Source: CAD feature listing. Evaluate the final solid. Frame: model axes, mm. A direction names the side the tool comes from. Coordinates: 2 decimals unless noted, no trailing zeros. Loops run counter-clockwise (first coordinate to the right, second up) from the corner with the lowest first, then second, coordinate; pieces in that order, holes last. Notation, with made-up numbers: (34.5, 3) -> (75.5, 3) arc R25 cw to (75.5, 19) -> close; hole circle Ø7 at (13, 19.25). An arc over 180 degrees is marked (long way). Answer as CSV lines item,"result".
from build123d import *

# Parameters (mm, degrees)
SKETCH1_W           = 260
SKETCH1_H           = 255
SKETCH1_R           = 60
BOSS_EXTRUDE1_DEPTH = 8
SKETCH2_W           = 315
SKETCH2_H           = 70
SKETCH2_W_2         = 80
SKETCH2_H_2         = 30
SKETCH2_W_3         = 70
BOSS_EXTRUDE2_DEPTH = 60
BOSS_EXTRUDE3_DEPTH = 60
CUT_EXTRUDE1_REACH  = 282.827
CUT_EXTRUDE2_REACH  = 282.827


with BuildPart() as part:
    # Sketch1 → Boss-Extrude1 (new body)
    with BuildSketch(Plane.XY):
        with Locations((130, 127.5)):
            Rectangle(SKETCH1_W, SKETCH1_H)
        with Locations((130, 145)):
            Circle(SKETCH1_R, mode=Mode.SUBTRACT)
    extrude(amount=BOSS_EXTRUDE1_DEPTH)

    # Sketch2 → Boss-Extrude2 (add)
    with BuildSketch(Plane.XY.offset(8)):
        with Locations((130, -35)):
            Rectangle(SKETCH2_W, SKETCH2_H)
        with Locations((40, -35)):
            Rectangle(SKETCH2_W_2, SKETCH2_H_2, mode=Mode.SUBTRACT)
        with Locations((220, -35)):
            Rectangle(SKETCH2_W_2, SKETCH2_H_2, mode=Mode.SUBTRACT)
        with Locations((130, -35)):
            Rectangle(SKETCH2_W_3, SKETCH2_H_2, mode=Mode.SUBTRACT)
    extrude(amount=-BOSS_EXTRUDE2_DEPTH)

    # Sketch3 → Boss-Extrude3 (add)
    with BuildSketch(Plane(origin=(0, 0, 0), x_dir=(1, 0, 0), z_dir=(0, 1, 0))):
        Polygon((260, -8), (287.5, 42), (284.121880998, 43.857965451), (260, 0), align=None)
        Polygon((0, -8), (-27.5, 42), (-24.121880998, 43.857965451), (0, 0), align=None)
    extrude(amount=BOSS_EXTRUDE3_DEPTH)

    # Sketch4 → Cut-Extrude1 (cut, up to next)
    with BuildSketch(Plane(origin=(202.994241843, 0, 111.646833013), x_dir=(0.48191875, 0, -0.876215909), z_dir=(0.876215909, 0, 0.48191875)), mode=Mode.PRIVATE) as cut_extrude1_sk1:
        Polygon((175.352708724, 0), (125.298874941, 60), (175.352708724, 60), align=None)
    cut_extrude1_tool1 = extrude(cut_extrude1_sk1.sketch, amount=-CUT_EXTRUDE1_REACH, mode=Mode.PRIVATE) & part.part
    add(cut_extrude1_tool1.solids().sort_by_distance((279.459373, 40, -27.380678))[0], mode=Mode.SUBTRACT)

    # Sketch5 → Cut-Extrude2 (cut, up to next)
    with BuildSketch(Plane(origin=(-3.378119002, 0, 1.857965451), x_dir=(0.48191875, 0, 0.876215909), z_dir=(-0.876215909, 0, 0.48191875)), mode=Mode.PRIVATE) as cut_extrude2_sk1:
        Polygon((-50.053833783, 0), (0, 60), (-50.053833783, 60), align=None)
    cut_extrude2_tool1 = extrude(cut_extrude2_sk1.sketch, amount=-CUT_EXTRUDE2_REACH, mode=Mode.PRIVATE) & part.part
    add(cut_extrude2_tool1.solids().sort_by_distance((-19.459373, 40, -27.380678))[0], mode=Mode.SUBTRACT)


solid = part.part
(1) Cut plane A-A (y = 145). Return the cut outline in (x, z), then the cut area to 3 significant figures.
Computed values:
outline,"(0, 0) -> (70, 0) -> (70, 8) -> (0, 8) -> close; (190, 0) -> (260, 0) -> (260, 8) -> (190, 8) -> close"
area,"1,120 mm^2"
(2) Material intervals for L1, parallel to Y at x = 130, z = 4; L2, parallel to Y at x = 75, z = -24; L3, parallel to Y at x = 232.5, z = 1, sorted ascending. Write a range as [from, to].
Computed values:
L1,"[-70, -50], [-20, 85], [205, 255]"
L2,"[-70, -50], [-20, 0]"
L3,"[-70, -50], [-20, 255]"
(3) Cut plane D-D (z = -27). Return the cut outline in (x, y).
Computed values:
outline,"(-27.5, -70) -> (287.5, -70) -> (287.5, 0) -> (279.25, 0) -> (279.25, 20.52) -> (274.85, 23.06) -> (274.85, 0) -> (-14.85, 0) -> (-14.85, 23.06) -> (-19.25, 20.52) -> (-19.25, 0) -> (-27.5, 0) -> close; hole (0, -50) -> (80, -50) -> (80, -20) -> (0, -20) -> close; hole (95, -50) -> (165, -50) -> (165, -20) -> (95, -20) -> close; hole (180, -50) -> (260, -50) -> (260, -20) -> (180, -20) -> close"
(4) Pin query (flat end, axial travel): pin 1 Ø6.5 at (y, z) = (204.5, 5.5) entering from +X; pin 2 Ø6 at (x, z) = (27, -29.5) entering from +Y; pin 3 Ø14 at (x, z) = (268, -25) entering from +Y. Return the tip coordinate at first contact, or that it passes through.
Computed values:
pin 1,"x = 260"
pin 2,"y = 0"
pin 3,"y = 34.95"
(5) Cut plane C-C (x = 205). Return the cut outline in (y, z), then the cut area to 3 significant figures.
Computed values:
outline,"(-70, -52) -> (-50, -52) -> (-50, 8) -> (-70, 8) -> close; (-20, -52) -> (0, -52) -> (0, 0) -> (255, 0) -> (255, 8) -> (-20, 8) -> close"
area,"4,440 mm^2"
(6) Cut plane B-B (x = 130). Return the cut outline in (y, z).
Computed values:
outline,"(-70, -52) -> (-50, -52) -> (-50, 8) -> (-70, 8) -> close; (-20, -52) -> (0, -52) -> (0, 0) -> (85, 0) -> (85, 8) -> (-20, 8) -> close; (205, 0) -> (255, 0) -> (255, 8) -> (205, 8) -> close"
(7) Draft query along Y for faces 4 (the flat face through (-10.5, 22.91, -11.09)), 5 (the flat face through (-13.9, 29.6, -21.3)), 6 (the flat face through (180, -35, -22)). Return one class per face: released by +Y, released by -Y, zero draft, split by the parting line, or undercut.
Computed values:
face 4,"zero draft"
face 5,"released by +Y"
face 6,"undercut"
(8) Access query for faces 1 (the flat face through (219, -20, -22)), 2 (the flat face through (280, 0, -6)), 3 (the flat face through (-6.87, 16.25, -12.49)). Directions: +Z, -Z, +X, -X, +Y, -Y. A direction counts if a zero-diameter tool reaches every point of the face in a straight line with its end or side. Return the directions, or none.
Computed values:
face 1,"+Z, -Z"
face 2,"+Z, +X, +Y"
face 3,"-Z, +Y"
